```python
from build123d import *

# Parameters (mm, degrees)
SKETCH1_W           = 12
SKETCH1_H           = 18
BOSS_EXTRUDE1_DEPTH = 5


with BuildPart() as part:
    # Sketch1 → Boss-Extrude1 (new body)
    with BuildSketch(Plane.XY):
        Polygon((-25, 60), (25, 60), (25, 55), (50, 55), (50, -55), (25, -55), (25, -60), (-25, -60), (-25, -55), (-50, -55), (-50, 55), (-25, 55), align=None)
        Polygon((37.651162791, 8), (42.651162791, 8), (42.651162791, -8), (37.651162791, -8), (37.651162791, -20), (8, -20), (8, -25), (-8, -25), (-8, -20), (-38.348837209, -20), (-38.348837209, -8), (-43.348837209, -8), (-43.348837209, 8), (-38.348837209, 8), (-38.348837209, 20), (-8, 20), (-8, 25), (8, 25), (8, 20), (37.651162791, 20), align=None, mode=Mode.SUBTRACT)
        with Locations((-32.348837209, 36)):
            Rectangle(SKETCH1_W, SKETCH1_H, mode=Mode.SUBTRACT)
    extrude(amount=BOSS_EXTRUDE1_DEPTH)


solid = part.part
```
Can you work these out from the model? Positions are in its coordinate system, mm. A direction names the side the tool comes from. Coordinates: 2 decimals unless noted, no trailing zeros. Loops run counter-clockwise (first coordinate to the right, second up) from the corner with the lowest first, then second, coordinate; pieces in that order, holes last. Notation, with made-up numbers: M -27,50.5 L -15,50.5 A7 cw -15,61.5 Z; hole C 71,42 d4. An arc over 180 degrees is marked long. Put each result on its own line as item: value. Start each with the question number.
(1) Which directions (+Z, -Z, +X, -X, +Y, -Y) give clear straight access to the entire face, cutting with the end or side of a thin tool? Please do faces 5 (the face through (37, 55, 2)), 6 (the face through (-38, 55, 2)), 7 (the face through (40, 8, 2)), 8 (the face through (-37, -55, 2)).
(2) Imagine slicing it at B-B on x = 34.5. List the corners of the cut face in (y, z) for me.
(3) Imagine slicing it at C-C on z = 3.1. Give the number of separate pieces and of enclosed holes in the cut face, and give its area (3 significant figures).
(4) I need wall thicknesses on probe 1 along X at (y, z) = (-17, 4.1); probe 2 along Y at (x, z) = (-39, 2.65); probe 3 along Y at (x, z) = (22.5, 3). Which ranges of each line are inside material? Lowest first, please.
(5) Imagine slicing it at A-A on y = -17. List the corners of the cut face in (x, z) for me, and give its area (3 significant figures).
(6) We'd pull the mould along X, two halves only. Please class faces 1 (the face through (0, -60, 2)), 2 (the face through (-43.349, 0, 2)), 3 (the face through (42.651, 0, 2)), 4 (the face through (-50, -1, 2)): +X half, -X half, draft (parallel to the pull), parting line (faces both ways), or undercut.
(7) Will these pins go through, and if not, where does the flat tip stop? pin 1 Ø3 at (x, y) = (16.5, -35) entering from -Z; pin 2 Ø2 at (x, z) = (-36, 1.5) entering from +Y.
Worked answers:
1. face 5: +Z, -Z, +X, +Y
1. face 6: +Z, -Z, -X, +Y
1. face 7: +Z, -Z
1. face 8: +Z, -Z, -X, -Y
2. outline: M -55,0 L -20,0 L -20,5 L -55,5 Z; M 20,0 L 55,0 L 55,5 L 20,5 Z
3. separate pieces: 1
3. enclosed holes: 2
3. area: 7,920 mm2
4. probe 1: x = -50 to -38.35, 37.65 to 50
4. probe 2: y = -55 to -8, 8 to 55
4. probe 3: y = -60 to -20, 20 to 60
5. outline: M -50,0 L -38.35,0 L -38.35,5 L -50,5 Z; M 37.65,0 L 50,0 L 50,5 L 37.65,5 Z
5. area: 120 mm2
6. face 1: draft
6. face 2: undercut
6. face 3: undercut
6. face 4: -X half
7. pin 1: stops at z = 0
7. pin 2: stops at y = 55
